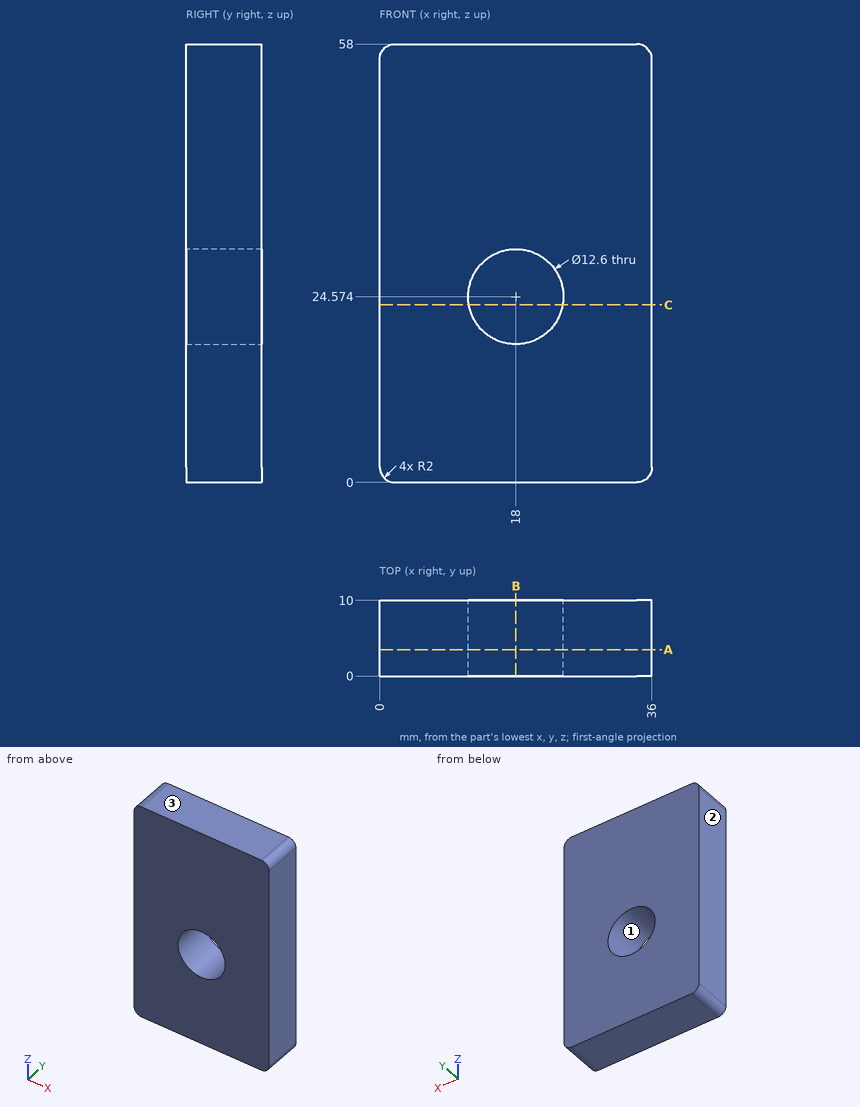
Study the drawing (mm; zero at the part's minimum x, y, z) and answer. Give positions to 0.01 mm unless a question says otherwise; leave off trailing zeros. Write each loop counter-clockwise with the first axis right and the second up, starting at its lowest first coordinate (ties: lowest second). Pieces come first, ordered by that corner, then holes. Notation, with made-up numbers: (57, 65) - (104, 65) arc R7 ccw to (104, 78) - close; hole circle Ø8 at (-22, -17.75). An arc over 180 degrees is marked (long way). Use a Markdown table: item, result.
1. Section A-A on y = 3.5 is taken. Write down the section's boundary in (x, z) (1 decimal), plus the area to 3 significant figures.
Values follow:
| item | result |
|---|---|
| outline | (0, 2) arc R2 ccw to (2, 0) - (34, 0) arc R2 ccw to (36, 2) - (36, 56) arc R2 ccw to (34, 58) - (2, 58) arc R2 ccw to (0, 56) - close; hole circle Ø12.6 at (18, 24.6) |
| area | 1,960 mm² |
2. Find the intervals of material crossed by probe 1 along X at (y, z) = (1, 27) (1 decimal); probe 2 along Z at (x, y) = (14.5, 5) (1 decimal); probe 3 along Z at (x, y) = (19, 2) (1 decimal), in increasing order. Write a range as from..to.
Values follow:
| item | result |
|---|---|
| probe 1 | x = 0..12.2, 23.8..36 |
| probe 2 | z = 0..19.3, 29.8..58 |
| probe 3 | z = 0..18.4, 30.8..58 |
3. Section C-C on z = 23.5 is taken. Write down the section's boundary in (x, y).
Values follow:
| item | result |
|---|---|
| outline | (0, 0) - (11.79, 0) - (11.79, 10) - (0, 10) - close; (24.21, 0) - (36, 0) - (36, 10) - (24.21, 10) - close |
4. Section B-B on x = 18 is taken. Write down the section's boundary in (y, z) (1 decimal).
Values follow:
| item | result |
|---|---|
| outline | (0, 0) - (10, 0) - (10, 18.3) - (0, 18.3) - close; (0, 30.9) - (10, 30.9) - (10, 58) - (0, 58) - close |
5. For a pull along Z with two mould halves and no side action, classify the marked faces 1, 2 and 3 as released by +Z, released by -Z, zero draft, split by the parting line, or undercut.
Values follow:
| item | result |
|---|---|
| face 1 | undercut |
| face 2 | zero draft |
| face 3 | released by +Z |
